Input: part model. Units: mm. Frame: model coordinates. A direction names the side the tool comes from. Round coordinates to 2 decimals unless told otherwise and drop trailing zeros. Loops run counter-clockwise (first coordinate to the right, second up) from the corner with the lowest first, then second, coordinate; pieces in that order, holes last. Notation, with made-up numbers: (14, 83) -> (70, 83) arc R34 cw to (70, 115) -> close; hole circle Ø7 at (86.5, 56). An arc over 180 degrees is marked (long way). Answer as a JSON object with one key per item and string values.
```python
from build123d import *

# Parameters (mm, degrees)
SKETCH1_W                    = 260
SKETCH1_H                    = 200
BASE_FLANGE1_DEPTH           = 5
EDGE_FLANGE1_STRIP_W         = 20.4
EDGE_FLANGE1_STRIP_H         = 5
EDGE_FLANGE1_STRIP_CUT_DEPTH = 260
EDGE_FLANGE1_DEPTH           = 260
EDGE_FLANGE2_STRIP_W         = 20.4
EDGE_FLANGE2_STRIP_H         = 5
EDGE_FLANGE2_STRIP_CUT_DEPTH = 260
EDGE_FLANGE2_DEPTH           = 260
CUT_EXTRUDE1_DEPTH           = 193.093727123
CUT_EXTRUDE1_DEPTH_BACK      = 193.093727123
SKETCH12_R                   = 40
CUT_EXTRUDE2_DEPTH           = 193.093727123
CUT_EXTRUDE2_DEPTH_BACK      = 193.093727123
SKETCH13_R                   = 9.5
CUT_EXTRUDE3_DEPTH           = 259.650343128
CUT_EXTRUDE3_DEPTH_BACK      = 259.650343128
SKETCH14_R                   = 7


# Sheet-metal steps are written as plain solids
with BuildPart() as part:
    # Sketch1 → Base-Flange1 (new body)
    with BuildSketch(Plane.XY):
        Rectangle(SKETCH1_W, SKETCH1_H)
    extrude(amount=-BASE_FLANGE1_DEPTH)

    # Edge-Flange1 strip (across the edge) → Edge-Flange1 strip cut (cut)
    with BuildSketch(Plane(origin=(-130, 100, -5), x_dir=(0, -1, 0), z_dir=(1, 0, 0))):
        with Locations((-5, -2.5)):
            Rectangle(EDGE_FLANGE1_STRIP_W, EDGE_FLANGE1_STRIP_H)
    extrude(amount=EDGE_FLANGE1_STRIP_CUT_DEPTH, mode=Mode.SUBTRACT)

    # Edge-Flange1 section (across the edge) → Edge-Flange1 (add)
    with BuildSketch(Plane(origin=(-130, 100, -5), x_dir=(0, -1, 0), z_dir=(1, 0, 0))):
        with BuildLine():
            Line((0, 0.2), (0, 95))
            Line((0, 95), (5, 95))
            Line((5, 95), (5, 0.2))
            ThreePointArc((5, 0.2), (5.058578644, 0.058578644), (5.2, 0))
            Line((5.2, 0), (5.2, -5))
            ThreePointArc((5.2, -5), (1.523044738, -3.476955262), (0, 0.2))
        make_face()
    extrude(amount=EDGE_FLANGE1_DEPTH)

    # Edge-Flange2 strip (across the edge) → Edge-Flange2 strip cut (cut)
    with BuildSketch(Plane(origin=(130, -100, -5), x_dir=(0, 1, 0), z_dir=(-1, 0, 0))):
        with Locations((-5, -2.5)):
            Rectangle(EDGE_FLANGE2_STRIP_W, EDGE_FLANGE2_STRIP_H)
    extrude(amount=EDGE_FLANGE2_STRIP_CUT_DEPTH, mode=Mode.SUBTRACT)

    # Edge-Flange2 section (across the edge) → Edge-Flange2 (add)
    with BuildSketch(Plane(origin=(130, -100, -5), x_dir=(0, 1, 0), z_dir=(-1, 0, 0))):
        with BuildLine():
            Line((0, 0.2), (0, 95))
            Line((0, 95), (5, 95))
            Line((5, 95), (5, 0.2))
            ThreePointArc((5, 0.2), (5.058578644, 0.058578644), (5.2, 0))
            Line((5.2, 0), (5.2, -5))
            ThreePointArc((5.2, -5), (1.523044738, -3.476955262), (0, 0.2))
        make_face()
    extrude(amount=EDGE_FLANGE2_DEPTH)

    # Sketch12 → Cut-Extrude1 (cut, two sides: drawn at the far end of the back side and taken through both)
    with BuildSketch(Plane.XY.offset(-CUT_EXTRUDE1_DEPTH_BACK)):
        with Locations(Location((0, 0, 0), (0, 0, 180))):
            Circle(SKETCH12_R)
    extrude(amount=CUT_EXTRUDE1_DEPTH + CUT_EXTRUDE1_DEPTH_BACK, mode=Mode.SUBTRACT)

    # Sketch13 → Cut-Extrude2 (cut, two sides: drawn at the far end of the back side and taken through both)
    with BuildSketch(Plane.XY.offset(-CUT_EXTRUDE2_DEPTH_BACK)):
        with Locations(Location((74.5, 74.5, 0), (0, 0, 180))):
            Circle(SKETCH13_R)
        with Locations(Location((-74.5, 74.5, 0), (0, 0, 180))):
            Circle(SKETCH13_R)
        with Locations(Location((-74.5, -74.5, 0), (0, 0, 180))):
            Circle(SKETCH13_R)
        with Locations(Location((74.5, -74.5, 0), (0, 0, 180))):
            Circle(SKETCH13_R)
    extrude(amount=CUT_EXTRUDE2_DEPTH + CUT_EXTRUDE2_DEPTH_BACK, mode=Mode.SUBTRACT)

    # Sketch14 → Cut-Extrude3 (cut, two sides: drawn at the far end of the back side and taken through both)
    with BuildSketch(Plane(origin=(0, -100, 0), x_dir=(-1, 0, 0), z_dir=(0, -1, 0)).offset(-CUT_EXTRUDE3_DEPTH_BACK)):
        with Locations(Location((110, 85, 0), (0, 0, 270))):
            Circle(SKETCH14_R)
        with Locations(Location((-110, 85, 0), (0, 0, 270))):
            Circle(SKETCH14_R)
    extrude(amount=CUT_EXTRUDE3_DEPTH + CUT_EXTRUDE3_DEPTH_BACK, mode=Mode.SUBTRACT)


solid = part.part
```
1) Section A-A, the plane y = -74.5. Output: boundary loops of the cut face in (x, z).
Output:
{"outline": "(-130, -5) -> (-84, -5) -> (-84, 0) -> (-130, 0) -> close; (-65, -5) -> (65, -5) -> (65, 0) -> (-65, 0) -> close; (84, -5) -> (130, -5) -> (130, 0) -> (84, 0) -> close"}
2) Contact query for a flat-ended pin moving along its axis: P1, Ø1, axis at x = 77, y = -58.5, coming from the -Z side. Output: stop coordinate, or through.
Output:
{"P1": "stops at z = -5"}
3) Section B-B, the plane x = 0. Output: boundary loops of the cut face in (y, z), plus the area to 3 significant figures.
Output:
{"outline": "(-100, -100) -> (-95, -100) -> (-95, -5.2) arc R0.2 cw to (-94.8, -5) -> (-40, -5) -> (-40, 0) -> (-94.8, 0) arc R5.2 ccw to (-100, -5.2) -> close; (40, -5) -> (94.8, -5) arc R0.2 cw to (95, -5.2) -> (95, -100) -> (100, -100) -> (100, -5.2) arc R5.2 ccw to (94.8, 0) -> (40, 0) -> close", "area": "1,540 mm^2"}
4) Ray query, probe 1 along X at (y, z) = (-98.4, -85); probe 2 along Y at (x, z) = (-34, -34); probe 3 along X at (y, z) = (-74, -2). Return the intervals inside material, ascending.
Output:
{"probe 1": "x = -130 to -117, -103 to 103, 117 to 130", "probe 2": "y = -100 to -95, 95 to 100", "probe 3": "x = -130 to -83.99, -65.01 to 65.01, 83.99 to 130"}
5) Section C-C, the plane z = -25. Output: boundary loops of the cut face in (x, y).
Output:
{"outline": "(-130, -100) -> (130, -100) -> (130, -95) -> (-130, -95) -> close; (-130, 95) -> (130, 95) -> (130, 100) -> (-130, 100) -> close"}
6) Reachability of faces 4 (the face through (2, -95, -53)), 5 (the face through (-110, 98, -92)) from +Z, -Z, +X, -X, +Y, -Y: full face, straight path, thin tool, end or side. Return the list, or none.
Output:
{"face 4": "-Z, +X, -X", "face 5": "+Y, -Y"}
7) Draft query along Z for faces 1 (the face through (110, 98, -92)), 2 (the face through (-2, -41, 0)), 3 (the face through (-79.61, -82.51, -2.53)). Return one class per face: +Z half, -Z half, draft (parallel to the pull), parting line (faces both ways), or undercut.
Output:
{"face 1": "undercut", "face 2": "+Z half", "face 3": "draft"}
8) Section D-D, the plane y = 0. Output: boundary loops of the cut face in (x, z).
Output:
{"outline": "(-130, -5) -> (-40, -5) -> (-40, 0) -> (-130, 0) -> close; (40, -5) -> (130, -5) -> (130, 0) -> (40, 0) -> close"}
